```python
from build123d import *

# Parameters (mm, degrees)
SKETCH1_W           = 635
SKETCH1_H           = 736.6
SKETCH1_W_2         = 584.2
SKETCH1_H_2         = 685.8
BOSS_EXTRUDE1_DEPTH = 50.8


with BuildPart() as part:
    # Sketch1 → Boss-Extrude1 (new body)
    # profile 1 of 13: a face of its own
    with BuildSketch(Plane(origin=(0, 0, 0), x_dir=(1, 0, 0), z_dir=(0, 1, 0))):
        Rectangle(SKETCH1_W, SKETCH1_H)
        Rectangle(SKETCH1_W_2, SKETCH1_H_2, mode=Mode.SUBTRACT)
    # profile 2 of 13: a face of its own
    with BuildSketch(Plane(origin=(0, 0, 0), x_dir=(1, 0, 0), z_dir=(0, 1, 0))):
        Polygon((176.657, -215.876084731), (49.633084731, -342.9), (85.554109215, -342.9), (292.1, -136.354109215), (292.1, -100.433084731), (215.9, -176.633084731), (202.057, -190.476084731), (190.5, -202.033084731), align=None)
    # profile 3 of 13: a face of its own
    with BuildSketch(Plane(origin=(0, 0, 0), x_dir=(1, 0, 0), z_dir=(0, 1, 0))):
        Polygon((85.554109215, 342.9), (49.633084731, 342.9), (176.657, 215.876084731), (190.5, 202.033084731), (202.057, 190.476084731), (215.9, 176.633084731), (292.1, 100.433084731), (292.1, 136.354109215), align=None)
    # profile 4 of 13: a face of its own
    with BuildSketch(Plane(origin=(0, 0, 0), x_dir=(1, 0, 0), z_dir=(0, 1, 0))):
        Polygon((-85.554109215, 342.9), (-292.1, 136.354109215), (-292.1, 100.433084731), (-215.9, 176.633084731), (-202.057, 190.476084731), (-190.5, 202.033084731), (-176.657, 215.876084731), (-49.633084731, 342.9), align=None)
    # profile 5 of 13: a face of its own
    with BuildSketch(Plane(origin=(0, 0, 0), x_dir=(1, 0, 0), z_dir=(0, 1, 0))):
        Polygon((-215.9, -176.633084731), (-292.1, -100.433084731), (-292.1, -136.354109215), (-85.554109215, -342.9), (-49.633084731, -342.9), (-176.657, -215.876084731), (-190.5, -202.033084731), (-202.057, -190.476084731), align=None)
    # profile 6 of 13: a face of its own
    with BuildSketch(Plane(origin=(0, 0, 0), x_dir=(1, 0, 0), z_dir=(0, 1, 0))):
        Polygon((176.657, 215.876084731), (-176.657, 215.876084731), (-190.5, 202.033084731), (-190.5, 190.476084731), (190.5, 190.476084731), (190.5, 202.033084731), align=None)
    # profile 7 of 13: a face of its own
    with BuildSketch(Plane(origin=(0, 0, 0), x_dir=(1, 0, 0), z_dir=(0, 1, 0))):
        Polygon((-202.057, 190.476084731), (-215.9, 176.633084731), (-215.9, -176.633084731), (-202.057, -190.476084731), (-190.5, -190.476084731), (-190.5, 190.476084731), align=None)
    # profile 8 of 13: a face of its own
    with BuildSketch(Plane(origin=(0, 0, 0), x_dir=(1, 0, 0), z_dir=(0, 1, 0))):
        Polygon((202.057, 190.476084731), (190.5, 190.476084731), (190.5, -190.476084731), (202.057, -190.476084731), (215.9, -176.633084731), (215.9, 176.633084731), align=None)
    # profile 9 of 13: a face of its own
    with BuildSketch(Plane(origin=(0, 0, 0), x_dir=(1, 0, 0), z_dir=(0, 1, 0))):
        Polygon((-190.5, -190.476084731), (-190.5, -202.033084731), (-176.657, -215.876084731), (176.657, -215.876084731), (190.5, -202.033084731), (190.5, -190.476084731), align=None)
    # profile 10 of 13: a face of its own
    with BuildSketch(Plane(origin=(0, 0, 0), x_dir=(1, 0, 0), z_dir=(0, 1, 0))):
        Polygon((-190.5, 202.033084731), (-202.057, 190.476084731), (-190.5, 190.476084731), align=None)
    # profile 11 of 13: a face of its own
    with BuildSketch(Plane(origin=(0, 0, 0), x_dir=(1, 0, 0), z_dir=(0, 1, 0))):
        Polygon((-190.5, -190.476084731), (-202.057, -190.476084731), (-190.5, -202.033084731), align=None)
    # profile 12 of 13: a face of its own
    with BuildSketch(Plane(origin=(0, 0, 0), x_dir=(1, 0, 0), z_dir=(0, 1, 0))):
        Polygon((202.057, -190.476084731), (190.5, -190.476084731), (190.5, -202.033084731), align=None)
    # profile 13 of 13: a face of its own
    with BuildSketch(Plane(origin=(0, 0, 0), x_dir=(1, 0, 0), z_dir=(0, 1, 0))):
        Polygon((202.057, 190.476084731), (190.5, 202.033084731), (190.5, 190.476084731), align=None)
    extrude(amount=BOSS_EXTRUDE1_DEPTH)


solid = part.part
```
The listing builds one solid part. Answer for the finished solid, in the listing's coordinates (mm). Round coordinates to 2 decimals unless told otherwise and drop trailing zeros. Loops run counter-clockwise (first coordinate to the right, second up) from the corner with the lowest first, then second, coordinate; pieces in that order, holes last.
Q1. Section C-C, the plane z = -149 is taken. Determine the outline of the cut face in (x, y).
Q2. Find the intervals of material crossed by line 1 (X direction, y = 47, z = 32); line 2 (Z direction, x = -0.5, y = 30); line 3 (Z direction, x = -93, y = 25.5), in increasing order.
Q3. For a pull along X with two mould halves and no side action, classify faces 1 (the face through (-4, 25, 368.3)), 2 (the face through (-190, 25, -342.9)) as released by +X, released by -X, zero draft, split by the parting line, or undercut.
Q4. Section A-A, the plane x = -26.5 is taken. Determine the outline of the cut face in (y, z).
Q5. Section D-D, the plane z = 203 is taken. Determine the outline of the cut face in (x, y).
Q6. Section B-B, the plane z = 23 is taken. Determine the outline of the cut face in (x, y), then the cut area to 3 significant figures.
Completed:
1. outline: (-317.5, 0) - (-292.1, 0) - (-292.1, 50.8) - (-317.5, 50.8) - close; (-279.45, 0) - (-243.53, 0) - (-243.53, 50.8) - (-279.45, 50.8) - close; (-215.9, 0) - (-190.5, 0) - (-190.5, 50.8) - (-215.9, 50.8) - close; (190.5, 0) - (215.9, 0) - (215.9, 50.8) - (190.5, 50.8) - close; (243.53, 0) - (279.45, 0) - (279.45, 50.8) - (243.53, 50.8) - close; (292.1, 0) - (317.5, 0) - (317.5, 50.8) - (292.1, 50.8) - close
2. line 1: x = -317.5 to -292.1, -215.9 to -190.5, 190.5 to 215.9, 292.1 to 317.5
2. line 2: z = -368.3 to -342.9, -215.88 to -190.48, 190.48 to 215.88, 342.9 to 368.3
2. line 3: z = -368.3 to -342.9, -335.45 to -299.53, -215.88 to -190.48, 190.48 to 215.88, 299.53 to 335.45, 342.9 to 368.3
3. face 1: zero draft
3. face 2: undercut
4. outline: (0, -368.3) - (50.8, -368.3) - (50.8, -342.9) - (0, -342.9) - close; (0, -215.88) - (50.8, -215.88) - (50.8, -190.48) - (0, -190.48) - close; (0, 190.48) - (50.8, 190.48) - (50.8, 215.88) - (0, 215.88) - close; (0, 342.9) - (50.8, 342.9) - (50.8, 368.3) - (0, 368.3) - close
5. outline: (-317.5, 0) - (-292.1, 0) - (-292.1, 50.8) - (-317.5, 50.8) - close; (-225.45, 0) - (225.45, 0) - (225.45, 50.8) - (-225.45, 50.8) - close; (292.1, 0) - (317.5, 0) - (317.5, 50.8) - (292.1, 50.8) - close
6. outline: (-317.5, 0) - (-292.1, 0) - (-292.1, 50.8) - (-317.5, 50.8) - close; (-215.9, 0) - (-190.5, 0) - (-190.5, 50.8) - (-215.9, 50.8) - close; (190.5, 0) - (215.9, 0) - (215.9, 50.8) - (190.5, 50.8) - close; (292.1, 0) - (317.5, 0) - (317.5, 50.8) - (292.1, 50.8) - close
6. area: 5,160 mm2
